```python
from build123d import *

# Parameters (mm, degrees)
F0_W     = 101.6
F0_H     = 101.6
F1_DEPTH = 50.8
F2_W     = 12.7
F2_H     = 69.85
F3_DEPTH = 50.8
F4_R     = 31.75
F5_DEPTH = 50.8


with BuildPart() as f1:
    # F0 (on Top) → F1 (new body, symmetric)
    with BuildSketch(Plane.XY):
        Rectangle(F0_W, F0_H)
    extrude(amount=F1_DEPTH, both=True)

    # F2 (on face) → F3 (cut)
    with BuildSketch(Plane.XY.offset(50.8)):
        with Locations((0, 1.10153)):
            Rectangle(F2_W, F2_H)
    extrude(amount=-F3_DEPTH, mode=Mode.SUBTRACT)

    # F4 (on face) → F5 (cut)
    with BuildSketch(Plane(origin=(-50.8, 0, 0), x_dir=(0, -1, 0), z_dir=(-1, 0, 0))):
        Circle(F4_R)
    extrude(amount=-F5_DEPTH, mode=Mode.SUBTRACT)


solid = f1.part
```
Geometry: final body of the model. Coordinates: model frame, mm. A direction names the side the tool comes from. Round coordinates to 2 decimals unless told otherwise and drop trailing zeros. Write each loop counter-clockwise with the first axis right and the second up, starting at its lowest first coordinate (ties: lowest second). Pieces come first, ordered by that corner, then holes.
Item 1: Section query A-A (y = 0). Return loops of the section in (x, z), plus the area to 3 significant figures.
Item 2: Pin query (flat end, axial travel): P1, Ø14, axis at x = 0, y = 12.5, coming from the +Z side; P2, Ø9.5, axis at y = 0.5, z = -20.5, coming from the -X side. Return the tip coordinate at first contact, or that it passes through.
Item 3: Section query B-B (x = -20). Return loops of the section in (y, z), plus the area to 3 significant figures.
Item 4: Section query D-D (y = 13). Return loops of the section in (x, z), plus the area to 3 significant figures.
Item 5: Section query C-C (z = 5). Return loops of the section in (x, y).
Item 6: Set-up query: faces 1 (the face through (11, 1, 50.8)), 2 (the face through (0, 0, -12)), 3 (the face through (0, -33.823, 26)). Return all of +Z, -Z, +X, -X, +Y, -Y with unobstructed straight access to the full face (end or side cutting, diameter ignored); none if empty.
Item 7: Material intervals for L1, parallel to Y at x = -15.5, z = 0; L2, parallel to Y at x = -6.5, z = -28, sorted ascending.
Item 8: Mould query, pull axis X, two halves, no side actions, for faces 4 (the face through (-25.756, 6.883, -30.995)), 5 (the face through (6.35, 1, 26)), 6 (the face through (50.8, -1, 1)). Classes: +X half, -X half, draft (parallel to the pull), parting line (faces both ways), or undercut.
Completed:
1. outline: (-50.8, -50.8) - (50.8, -50.8) - (50.8, 50.8) - (6.35, 50.8) - (6.35, 0) - (0, 0) - (0, -31.75) - (-50.8, -31.75) - close; (-50.8, 31.75) - (-6.35, 31.75) - (-6.35, 50.8) - (-50.8, 50.8) - close
1. area: 6,650 mm2
2. P1: stops at z = 50.8
2. P2: stops at x = 0
3. outline: (-50.8, -50.8) - (50.8, -50.8) - (50.8, 50.8) - (-50.8, 50.8) - close; hole circle Ø63.5 at (0, 0)
3. area: 7,160 mm2
4. outline: (-50.8, -50.8) - (50.8, -50.8) - (50.8, 50.8) - (6.35, 50.8) - (6.35, 0) - (0, 0) - (0, -28.97) - (-50.8, -28.97) - close; (-50.8, 28.97) - (-6.35, 28.97) - (-6.35, 50.8) - (-50.8, 50.8) - close
4. area: 6,920 mm2
5. outline: (-50.8, -50.8) - (50.8, -50.8) - (50.8, 50.8) - (-50.8, 50.8) - (-50.8, 31.35) - (-6.35, 31.35) - (-6.35, 36.03) - (6.35, 36.03) - (6.35, -33.82) - (-6.35, -33.82) - (-6.35, -31.35) - (-50.8, -31.35) - close
6. face 1: +Z, +X, -X, +Y, -Y
6. face 2: +Z, -X
6. face 3: +Z
7. L1: y = -50.8 to -31.75, 31.75 to 50.8
7. L2: y = -50.8 to -14.97, 14.97 to 50.8
8. face 4: draft
8. face 5: undercut
8. face 6: +X half
